Design review of the part built by this model. Coordinates are the model's own, in mm. Give positions to 0.01 mm unless a question says otherwise; leave off trailing zeros. Order: outer loops, then holes, each group sorted by start corner. A loop starts at its lowest first (then second) coordinate and runs counter-clockwise, first axis right, second up. Notation, with made-up numbers: M 83.25,1 L 90.25,1 A11 ccw 90.25,10 Z; hole C -12.5,-4.75 d7. An arc over 180 degrees is marked long. Put each result on its own line as item: value. Start each with the question number.
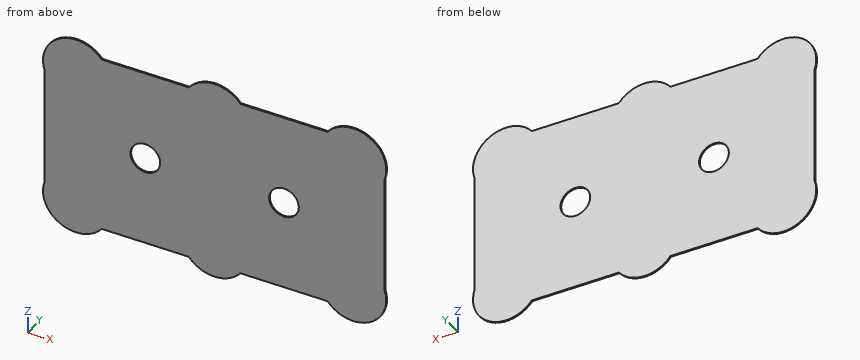
from build123d import *

# Parameters (mm, degrees)
SKETCH1_R           = 2.25
BOSS_EXTRUDE1_DEPTH = 0.2


with BuildPart() as part:
    # Sketch1 → Boss-Extrude1 (new body)
    with BuildSketch(Plane(origin=(0, 0, 0), x_dir=(1, 0, 0), z_dir=(0, 1, 0))):
        with BuildLine():
            Line((0.25, 24.4087505), (0.25, 6.5612495))
            ThreePointArc((0.25, 6.5612495), (2.618921791, 0.603357354), (8.903123749, 1.875))
            Line((8.903123749, 1.875), (22.096876251, 1.875))
            ThreePointArc((22.096876251, 1.875), (26, 0), (29.903123749, 1.875))
            Line((29.903123749, 1.875), (43.096876251, 1.875))
            ThreePointArc((43.096876251, 1.875), (49.381078209, 0.603357354), (51.75, 6.5612495))
            Line((51.75, 6.5612495), (51.75, 24.4087505))
            ThreePointArc((51.75, 24.4087505), (49.381078209, 30.366642646), (43.096876251, 29.095))
            Line((43.096876251, 29.095), (29.903123749, 29.095))
            ThreePointArc((29.903123749, 29.095), (26, 30.97), (22.096876251, 29.095))
            Line((22.096876251, 29.095), (8.903123749, 29.095))
            ThreePointArc((8.903123749, 29.095), (2.618921791, 30.366642646), (0.25, 24.4087505))
        make_face()
        with Locations((15.5, 15.485)):
            Circle(SKETCH1_R, mode=Mode.SUBTRACT)
        with Locations((36.5, 15.485)):
            Circle(SKETCH1_R, mode=Mode.SUBTRACT)
    extrude(amount=BOSS_EXTRUDE1_DEPTH)


solid = part.part
1. Consider section C-C on z = -15. Give the boundary of the cut face in (x, y).
2. Consider section B-B on y = 0.05. Give the boundary of the cut face in (x, z) (3 decimals).
3. Consider section A-A on x = 36.5. Give the boundary of the cut face in (y, z) (3 decimals), then the cut area to 3 significant figures.
4. To check wall thickness, follow probe 1 along Z at (x, y) = (36.5, 0.15) (3 decimals); probe 2 along X at (y, z) = (0.1, -1.5); probe 3 along X at (y, z) = (0.1, -27.5). State the ranges of each line that lie inside material, in increasing order.
5. Consider section D-D on x = 15. Give the boundary of the cut face in (y, z) (3 decimals), then the cut area to 3 significant figures.
Returned:
1. outline: M 0.25,0 L 13.3,0 L 13.3,0.2 L 0.25,0.2 Z; M 17.7,0 L 34.3,0 L 34.3,0.2 L 17.7,0.2 Z; M 38.7,0 L 51.75,0 L 51.75,0.2 L 38.7,0.2 Z
2. outline: M 0.25,-24.409 A5 ccw 8.903,-29.095 L 22.097,-29.095 A5 ccw 29.903,-29.095 L 43.097,-29.095 A5 ccw 51.75,-24.409 L 51.75,-6.561 A5 ccw 43.097,-1.875 L 29.903,-1.875 A5 ccw 22.097,-1.875 L 8.903,-1.875 A5 ccw 0.25,-6.561 Z; hole C 15.5,-15.485 d4.5; hole C 36.5,-15.485 d4.5
3. outline: M 0,-29.095 L 0.2,-29.095 L 0.2,-17.735 L 0,-17.735 Z; M 0,-13.235 L 0.2,-13.235 L 0.2,-1.875 L 0,-1.875 Z
3. area: 4.54 mm2
4. probe 1: z = -29.095 to -17.735, -13.235 to -1.875
4. probe 2: x = 1.43 to 8.57, 22.43 to 29.57, 43.43 to 50.57
4. probe 3: x = 0.24 to 51.76
5. outline: M 0,-29.095 L 0.2,-29.095 L 0.2,-17.679 L 0,-17.679 Z; M 0,-13.291 L 0.2,-13.291 L 0.2,-1.875 L 0,-1.875 Z
5. area: 4.57 mm2
